Input: part model. Units: mm. Frame: model coordinates. A direction names the side the tool comes from. Coordinates: 2 decimals unless noted, no trailing zeros. Write each loop counter-clockwise with the first axis right and the second up, starting at its lowest first coordinate (ties: lowest second). Pieces come first, ordered by that corner, then holes. Notation, with made-up numbers: (66.25, 11.5) - (87.25, 11.5) arc R13 ccw to (87.25, 18.5) - close; hole circle Ø7 at (8.25, 80). An arc over 180 degrees is marked (long way). Use a Markdown table: item, result. Add a question column.
Q1. Pin query (flat end, axial travel): P1, Ø5, axis at y = -6.5, z = 6, coming from the +X side; P2, Ø5, axis at y = -170.5, z = 3.5, coming from the -X side; P3, Ø3, axis at x = 4, z = 4, coming from the -Y side. Return the tip coordinate at first contact, or that it passes through.
Q2. Set-up query: faces 1 (the face through (173, -120.65, 5)), 2 (the face through (158.75, -173, 5)), 3 (the face through (15, -167.386, 5)). Return all of +Z, -Z, +X, -X, +Y, -Y with unobstructed straight access to the full face (end or side cutting, diameter ignored); none if empty.
Q3. Section query C-C (y = -144). Return the cut outline in (x, z).
Q4. Mould query, pull axis X, two halves, no side actions, for faces 4 (the face through (31.75, -5, 5)), 5 (the face through (167.386, -163, 5)), 6 (the face through (0, -25, 5)), 7 (the face through (173, -146.05, 5)). Classes: released by +X, released by -X, zero draft, split by the parting line, or undercut.
Q5. Section query D-D (x = 165). Return the cut outline in (y, z), then the cut area to 3 significant figures.
Q6. Section query A-A (x = 89). Return the cut outline in (y, z), then the cut area to 3 significant figures.
Q7. Material intervals for probe 1 along Y at (x, z) = (7.5, 5.75); probe 2 along Y at (x, z) = (89, 4.75); probe 3 along Y at (x, z) = (101.5, 2.5), sorted ascending. Write a range as from..to.
Q8. Section query B-B (x = 129.5). Return the cut outline in (y, z), then the cut area to 3 significant figures.
from build123d import *

# Parameters (mm, degrees)
F1_DEPTH = 10.414


with BuildPart() as f1:
    # F0 (on Top) → F1 (new body)
    with BuildSketch(Plane.XY):
        Polygon((31.75, 0), (19.05, 0), (19.05, -10.414), (10.414, -10.414), (10.414, -19.05), (0, -19.05), (0, -31.75), (10.414, -31.75), (10.414, -44.45), (0, -44.45), (0, -57.15), (10.414, -57.15), (10.414, -69.85), (0, -69.85), (0, -82.55), (10.414, -82.55), (10.414, -95.25), (0, -95.25), (0, -107.95), (10.414, -107.95), (10.414, -120.65), (0, -120.65), (0, -133.35), (10.414, -133.35), (10.414, -146.05), (0, -146.05), (0, -158.75), (10.414, -158.75), (10.414, -167.386), (19.05, -167.386), (19.05, -177.8), (31.75, -177.8), (31.75, -167.386), (44.45, -167.386), (44.45, -177.8), (57.15, -177.8), (57.15, -167.386), (69.85, -167.386), (69.85, -177.8), (82.55, -177.8), (82.55, -167.386), (95.25, -167.386), (95.25, -177.8), (107.95, -177.8), (107.95, -167.386), (120.65, -167.386), (120.65, -177.8), (133.35, -177.8), (133.35, -167.386), (146.05, -167.386), (146.05, -177.8), (158.75, -177.8), (158.75, -167.386), (167.386, -167.386), (167.386, -158.75), (177.8, -158.75), (177.8, -146.05), (167.386, -146.05), (167.386, -133.35), (177.8, -133.35), (177.8, -120.65), (167.386, -120.65), (167.386, -107.95), (177.8, -107.95), (177.8, -95.25), (167.386, -95.25), (167.386, -82.55), (177.8, -82.55), (177.8, -69.85), (167.386, -69.85), (167.386, -57.15), (177.8, -57.15), (177.8, -44.45), (167.386, -44.45), (167.386, -31.75), (177.8, -31.75), (177.8, -19.05), (167.386, -19.05), (167.386, -10.414), (158.75, -10.414), (158.75, 0), (146.05, 0), (146.05, -10.414), (133.35, -10.414), (133.35, 0), (120.65, 0), (120.65, -10.414), (107.95, -10.414), (107.95, 0), (95.25, 0), (95.25, -10.414), (82.55, -10.414), (82.55, 0), (69.85, 0), (69.85, -10.414), (57.15, -10.414), (57.15, 0), (44.45, 0), (44.45, -10.414), (31.75, -10.414), align=None)
        with BuildLine():
            ThreePointArc((31.75, -69.596), (33.609872, -65.105872), (38.1, -63.246))
            Line((38.1, -63.246), (139.7, -63.246))
            ThreePointArc((139.7, -63.246), (144.190128, -65.105872), (146.05, -69.596))
            Line((146.05, -69.596), (146.05, -80.391))
            ThreePointArc((146.05, -80.391), (144.190128, -84.881128), (139.7, -86.741))
            Line((139.7, -86.741), (38.1, -86.741))
            ThreePointArc((38.1, -86.741), (33.609872, -84.881128), (31.75, -80.391))
            Line((31.75, -80.391), (31.75, -69.596))
        make_face(mode=Mode.SUBTRACT)
    extrude(amount=F1_DEPTH)


solid = f1.part
Values follow:
| question | item | result |
|---|---|---|
| 1 | P1 | x = 158.75 |
| 1 | P2 | x = 19.05 |
| 1 | P3 | y = -158.75 |
| 2 | face 1 | +Z, -Z, +X |
| 2 | face 2 | +Z, -Z, +X, -Y |
| 2 | face 3 | +Z, -Z, -X, -Y |
| 3 | outline | (10.41, 0) - (167.39, 0) - (167.39, 10.41) - (10.41, 10.41) - close |
| 4 | face 4 | undercut |
| 4 | face 5 | released by +X |
| 4 | face 6 | released by -X |
| 4 | face 7 | zero draft |
| 5 | outline | (-167.39, 0) - (-10.41, 0) - (-10.41, 10.41) - (-167.39, 10.41) - close |
| 5 | area | 1,630 mm2 |
| 6 | outline | (-167.39, 0) - (-86.74, 0) - (-86.74, 10.41) - (-167.39, 10.41) - close; (-63.25, 0) - (-10.41, 0) - (-10.41, 10.41) - (-63.25, 10.41) - close |
| 6 | area | 1,390 mm2 |
| 7 | probe 1 | -158.75..-146.05, -133.35..-120.65, -107.95..-95.25, -82.55..-69.85, -57.15..-44.45, -31.75..-19.05 |
| 7 | probe 2 | -167.39..-86.74, -63.25..-10.41 |
| 7 | probe 3 | -177.8..-86.74, -63.25..0 |
| 8 | outline | (-177.8, 0) - (-86.74, 0) - (-86.74, 10.41) - (-177.8, 10.41) - close; (-63.25, 0) - (0, 0) - (0, 10.41) - (-63.25, 10.41) - close |
| 8 | area | 1,610 mm2 |
